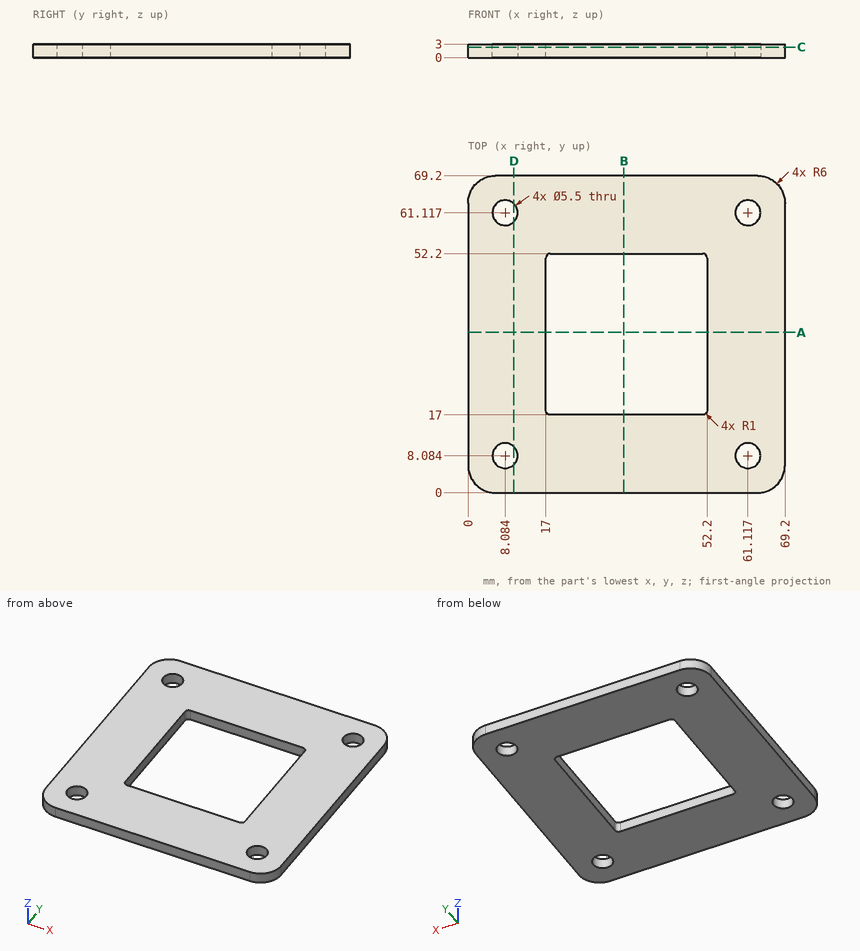
Check sheet for the drawn part. Datum: minimum x, y, z corner. Units: mm. Round coordinates to 2 decimals unless told otherwise and drop trailing zeros. Loops run counter-clockwise (first coordinate to the right, second up) from the corner with the lowest first, then second, coordinate; pieces in that order, holes last. Notation, with made-up numbers: (80.25, -16.75) -> (106.25, -16.75) arc R29 ccw to (106.25, 8.25) -> close; hole circle Ø9 at (62, 36.25). An arc over 180 degrees is marked (long way). Put each result on its own line as item: value. Start each with the question number.
1. Section check A-A (y = 35). Enter the section's corners in (x, z).
2. Section check D-D (x = 10). Enter the section's corners in (y, z) (1 decimal), plus the area to 3 significant figures.
3. Section check C-C (z = 2.3). Enter the section's corners in (x, y).
4. Scan lines: probe 1 along X at (y, z) = (40, 2.35); probe 2 along Y at (x, z) = (61, 1.75) (1 decimal). Record each from-to range of solid material in increasing order.
Findings:
1. outline: (0, 0) -> (17, 0) -> (17, 3) -> (0, 3) -> close; (52.2, 0) -> (69.2, 0) -> (69.2, 3) -> (52.2, 3) -> close
2. outline: (0, 0) -> (6.1, 0) -> (6.1, 3) -> (0, 3) -> close; (10.1, 0) -> (59.1, 0) -> (59.1, 3) -> (10.1, 3) -> close; (63.1, 0) -> (69.2, 0) -> (69.2, 3) -> (63.1, 3) -> close
2. area: 184 mm^2
3. outline: (0, 6) arc R6 ccw to (6, 0) -> (63.2, 0) arc R6 ccw to (69.2, 6) -> (69.2, 63.2) arc R6 ccw to (63.2, 69.2) -> (6, 69.2) arc R6 ccw to (0, 63.2) -> close; hole circle Ø5.5 at (8.08, 8.08); hole circle Ø5.5 at (8.08, 61.12); hole (17, 18) arc R1 ccw to (18, 17) -> (51.2, 17) arc R1 ccw to (52.2, 18) -> (52.2, 51.2) arc R1 ccw to (51.2, 52.2) -> (18, 52.2) arc R1 ccw to (17, 51.2) -> close; hole circle Ø5.5 at (61.12, 8.08); hole circle Ø5.5 at (61.12, 61.12)
4. probe 1: x = 0 to 17, 52.2 to 69.2
4. probe 2: y = 0 to 5.3, 10.8 to 58.4, 63.9 to 69.2
